Here's how the part is built. I have some questions about the finished solid (model axes, mm). A direction names the side the tool comes from. Round coordinates to 2 decimals unless told otherwise and drop trailing zeros. Write each loop counter-clockwise with the first axis right and the second up, starting at its lowest first coordinate (ties: lowest second). Pieces come first, ordered by that corner, then holes. Notation, with made-up numbers: M 80.25,87 L 96.25,87 A22 ccw 96.25,116 Z; hole C 24,68 d7. An arc over 180 degrees is marked long. Use one line per item in the form item = value. Start each with the question number.
Q1. I need wall thicknesses on line 1 along Y through (x, z) = (0, 27); line 2 along X through (y, z) = (-9.5, 32.5); line 3 along X through (y, z) = (22, 37). Which ranges of each line are inside material? Lowest first, please. Write a range as from..to.
Q2. For faces 1 (the face through (-26.3, -12.8, 4.9)), 2 (the face through (23, -10, 25)), 3 (the face through (-35.639, -9.812, 4.93)), 4 (the face through (17.32, 32.4, 4.93)), which set-ups out of +Z, -Z, +X, -X, +Y, -Y let a thin tool reach every point of the face, with its end or its side?
Q3. I want a section at D-D on z = 19. List the corners of the cut face in (x, y) for me, and give its area (3 significant figures).
Q4. I'm going to push flat-ended pins straight in: pin 1 Ø12 at (y, z) = (-35.5, 10) entering from -X; pin 2 Ø5 at (x, y) = (23.1, 9.57) entering from -Z; pin 3 Ø3 at (x, z) = (-26.5, 9.5) entering from +Y. Where does each tip first touch, or does it pass through?
Q5. I want a section at A-A on y = 0. List the corners of the cut face in (x, z) for me, and give its area (3 significant figures).
Q6. We'd pull the mould along X, two halves only. Please class faces 5 (the face through (23, 27, 0)), 6 (the face through (27.85, 24.3, 4.93)), 7 (the face through (15.48, 20.07, 32.61)): +X half, -X half, draft (parallel to the pull), parting line (faces both ways), or undercut.
Q7. I want a section at C-C on x = 0. List the corners of the cut face in (y, z) for me, and give its area (3 significant figures).
Q8. I want a section at B-B on z = 3. List the corners of the cut face in (x, y) for me.
```python
from build123d import *

# Parameters (mm, degrees)
SKETCH_R              = 45
PAD_DEPTH             = 40
SKETCH001_R           = 12
POCKET_DEPTH          = 40.001
SKETCH002_R           = 29.25
POCKET001_DEPTH       = 10
SKETCH003_R           = 3.25
POCKET002_DEPTH       = 15
POLARPATTERN_COUNT    = 16
SKETCH004_R           = 16
POCKET003_DEPTH       = 40.001
POCKET004_DEPTH       = 10
POLARPATTERN001_COUNT = 7


with BuildPart() as part:
    # Sketch → Pad (new body)
    with BuildSketch(Plane.XY):
        Circle(SKETCH_R)
    extrude(amount=PAD_DEPTH)

    # Sketch001 → Pocket (cut, through all)
    with BuildSketch(Plane(origin=(0, 0, 0), x_dir=(1, 0, 0), z_dir=(0, 0, -1))):
        Circle(SKETCH001_R)
    extrude(amount=-POCKET_DEPTH, mode=Mode.SUBTRACT)

    # Sketch002 → Pocket001 (cut)
    with BuildSketch(Plane(origin=(0, 0, 0), x_dir=(1, 0, 0), z_dir=(0, 0, -1))):
        Circle(SKETCH002_R)
    extrude(amount=-POCKET001_DEPTH, mode=Mode.SUBTRACT)

    # Sketch003 → Pocket002 (cut)
    with BuildSketch(Plane.XY.offset(40)):
        with Locations((0, 25)):
            Circle(SKETCH003_R)
    pocket002 = extrude(amount=-POCKET002_DEPTH, mode=Mode.SUBTRACT)

    # PolarPattern: Pocket002 ×16 about axis
    polarpattern_axis = Axis((0, 0, 40), (0, 0, 1))
    for i in range(1, POLARPATTERN_COUNT):
        add(pocket002.rotate(polarpattern_axis, i * 360 / POLARPATTERN_COUNT), mode=Mode.SUBTRACT)

    # Sketch004 → Pocket003 (cut, through all)
    with BuildSketch(Plane.XY.offset(40)):
        Circle(SKETCH004_R)
    extrude(amount=-POCKET003_DEPTH, mode=Mode.SUBTRACT)

    # Sketch005 → Pocket004 (cut)
    with BuildSketch(Plane(origin=(0, 0, 0), x_dir=(1, 0, 0), z_dir=(0, 0, -1))):
        Polygon((-12.266942, 54.255708), (34.539446, 43.617943), (8.189071, 26.52432), (11.054546, 21.833583), (-0.504584, 24.460645), (4.106836, 27.452097), align=None)
    pocket004 = extrude(amount=-POCKET004_DEPTH, mode=Mode.SUBTRACT)

    # PolarPattern001: Pocket004 ×7 about axis
    polarpattern001_axis = Axis((0, 0, 0), (0, 0, -1))
    for i in range(1, POLARPATTERN001_COUNT):
        add(pocket004.rotate(polarpattern001_axis, i * 360 / POLARPATTERN001_COUNT), mode=Mode.SUBTRACT)


solid = part.part
```
Reported:
q1.line_1 = -45..-28.25, -21.75..-16, 16..21.75, 28.25..45
q1.line_2 = -43.99..-26.35, -19.85..-12.87, 12.87..19.85, 26.35..43.99
q1.line_3 = -39.26..-12.63, -6.51..-1.25, 1.25..6.51, 12.63..39.26
q2.face_1 = -Z
q2.face_2 = +Z
q2.face_3 = -Z, -X
q2.face_4 = -Z, +Y
q3.outline = C 0,0 d90; hole C 0,0 d32
q3.area = 5,560 mm^2
q4.pin_1 = -33.98
q4.pin_2 = 10
q4.pin_3 = 37.36
q5.outline = M -45,10 L -16,10 L -16,40 L -21.75,40 L -21.75,25 L -28.25,25 L -28.25,40 L -45,40 Z; M 16,10 L 29.25,10 L 29.25,0 L 45,0 L 45,40 L 28.25,40 L 28.25,25 L 21.75,25 L 21.75,40 L 16,40 Z
q5.area = 1,700 mm^2
q6.face_5 = draft
q6.face_6 = +X half
q6.face_7 = undercut
q7.outline = M -45,10 L -34.17,10 L -34.17,0 L -29.25,0 L -29.25,10 L -16,10 L -16,40 L -21.75,40 L -21.75,25 L -28.25,25 L -28.25,40 L -45,40 Z; M 16,10 L 29.25,10 L 29.25,0 L 34.24,0 L 34.24,10 L 45,10 L 45,40 L 28.25,40 L 28.25,25 L 21.75,25 L 21.75,40 L 16,40 Z
q7.area = 1,640 mm^2
q8.outline = M -42.05,-16.04 A45 ccw -38.78,-22.82 L -20.8,-20.57 A29.25 cw -29.05,-3.41 Z; M -42.02,16.09 L -29.05,3.44 A29.25 cw -20.78,20.59 L -38.75,22.87 A45 ccw Z; M -15.45,-24.84 L -13.68,-42.87 A45 ccw -6.34,-44.55 L 3.11,-29.08 A29.25 cw Z; M -15.42,24.85 A29.25 cw 3.14,29.08 L -6.28,44.56 A45 ccw -13.62,42.89 Z; M 9.79,-27.56 L 24.99,-37.42 A45 ccw 30.88,-32.73 L 24.68,-15.7 A29.25 cw Z; M 9.82,27.55 A29.25 cw 24.69,15.68 L 30.92,32.69 A45 ccw 25.04,37.39 Z; M 27.65,-9.53 L 44.84,-3.79 A45 ccw 44.84,3.73 L 27.66,9.5 A29.25 cw Z
